Source: three-view drawing plus pictorial views. Frame: mm from the lowest corner of the part. A direction names the side the tool comes from. Give positions to 0.01 mm unless a question says otherwise; leave off trailing zeros. Loops run counter-clockwise (first coordinate to the right, second up) from the corner with the lowest first, then second, coordinate; pieces in that order, holes last. Notation, with made-up numbers: M 9,87.25 L 58,87.25 A24 cw 58,124.25 Z; hole C -27.5,31.5 d3. An arc over 180 degrees is marked long. Write item = value, one per line.
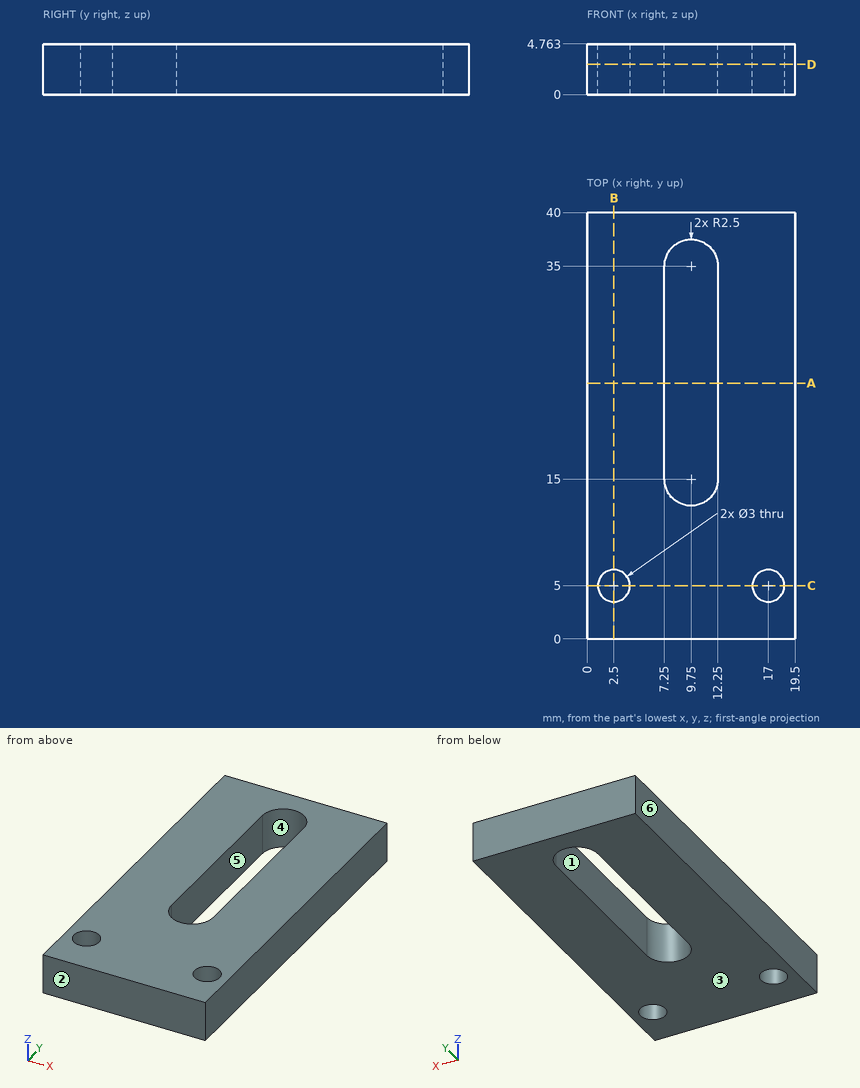
1. Cut plane D-D, the plane z = 2.85. Return the cut outline in (x, y).
Derived:
outline = M 0,0 L 19.5,0 L 19.5,40 L 0,40 Z; hole C 2.5,5 d3; hole M 7.25,15 A2.5 ccw 12.25,15 L 12.25,35 A2.5 ccw 7.25,35 Z; hole C 17,5 d3
2. Cut plane A-A, the plane y = 24. Return the cut outline in (x, z).
Derived:
outline = M 0,0 L 7.25,0 L 7.25,4.76 L 0,4.76 Z; M 12.25,0 L 19.5,0 L 19.5,4.76 L 12.25,4.76 Z
3. Cut plane B-B, the plane x = 2.5. Return the cut outline in (y, z).
Derived:
outline = M 0,0 L 3.5,0 L 3.5,4.76 L 0,4.76 Z; M 6.5,0 L 40,0 L 40,4.76 L 6.5,4.76 Z
4. Material intervals for probe 1 along X at (y, z) = (5, 2.8); probe 2 along X at (y, z) = (20.5, 2.3); probe 3 along Y at (x, z) = (17, 1.3), sorted ascending. Write a range as from..to.
Derived:
probe_1 = 0..1, 4..15.5, 18.5..19.5
probe_2 = 0..7.25, 12.25..19.5
probe_3 = 0..3.5, 6.5..40
5. Reachability of the marked faces 5 and 6 from +Z, -Z, +X, -X, +Y, -Y: full face, straight path, thin tool, end or side. Return the list, or none.
Derived:
face_5 = +Z, -Z
face_6 = +Z, -Z, -X, +Y, -Y
6. Cut plane C-C, the plane y = 5. Return the cut outline in (x, z).
Derived:
outline = M 0,0 L 1,0 L 1,4.76 L 0,4.76 Z; M 4,0 L 15.5,0 L 15.5,4.76 L 4,4.76 Z; M 18.5,0 L 19.5,0 L 19.5,4.76 L 18.5,4.76 Z
7. Pull-direction query (Y, two-part tool) for the marked faces 1, 2, 3 and 4; classes: +Y half, -Y half, draft (parallel to the pull), parting line (faces both ways), or undercut.
Derived:
face_1 = undercut
face_2 = -Y half
face_3 = draft
face_4 = undercut
8. First-contact query: pin 1 Ø2 at (x, z) = (10, 0.5) entering from -Y; pin 2 Ø1.8 at (x, y) = (17, 5) entering from -Z. Flat tips, straight axial feed; report the tip coordinate or a pass-through.
Derived:
pin_1 = 0
pin_2 = through
